Autodesk Inventor part; units mm, degrees
ref_plane "YZ Plane" through (0, 0, 0) normal (1, 0, 0) x (0, 1, 0)
ref_plane "XZ Plane" through (0, 0, 0) normal (0, 1, 0) x (-1, 0, 0)
ref_plane "XY Plane" through (0, 0, 0) normal (0, 0, 1) x (1, 0, 0)
sketch "Sketch1" plane through (0, 0, 0) normal (0, 0, 1) x (1, 0, 0)
  line L0 (0, 110) -> (110, 110)
  line L1 (110, 60) -> (110, 0)
  line L2 (110, 0) -> (0, 0)
  line L3 (0, 0) -> (0, 110)
  arc A0 (110, 110) -> (110, 60) centre (110, 85) ccw
  line L4 (73.8274, 98.9712) -> (73.8274, 60) construction
  line L5 (73.8274, 60) -> (92, 60) construction
  line L6 (73.8274, 98.9712) -> (92, 60)
  line L7 (92, 60) -> (73.8274, 98.9712) construction
  line L8 (73.8274, 98.9712) -> (71.1085, 97.7034)
  line L9 (71.1085, 97.7034) -> (89.2811, 58.7321)
  line L10 (89.2811, 58.7321) -> (92, 60)
  line L11 (0, 0) -> (10, 0)
  line L12 (10, 0) -> (10, -3)
  line L13 (10, -3) -> (0, -3)
  line L14 (0, -3) -> (0, 0)
  line L15 (30, 0) -> (30, -3)
  line L16 (20, 0) -> (30, 0)
  line L17 (20, -3) -> (20, 0)
  line L18 (30, -3) -> (20, -3)
  line L19 (50, 0) -> (50, -3)
  line L20 (40, 0) -> (50, 0)
  line L21 (40, -3) -> (40, 0)
  line L22 (50, -3) -> (40, -3)
  line L23 (70, 0) -> (70, -3)
  line L24 (60, 0) -> (70, 0)
  line L25 (60, -3) -> (60, 0)
  line L26 (70, -3) -> (60, -3)
  line L27 (90, 0) -> (90, -3)
  line L28 (80, 0) -> (90, 0)
  line L29 (80, -3) -> (80, 0)
  line L30 (90, -3) -> (80, -3)
  line L31 (110, 0) -> (110, -3)
  line L32 (100, 0) -> (110, 0)
  line L33 (100, -3) -> (100, 0)
  line L34 (110, -3) -> (100, -3)
  line L35 (10, 113) -> (10, 110)
  line L36 (0, 113) -> (10, 113)
  line L37 (0, 110) -> (0, 113)
  line L38 (10, 110) -> (0, 110)
  line L39 (30, 113) -> (30, 110)
  line L40 (20, 113) -> (30, 113)
  line L41 (20, 110) -> (20, 113)
  line L42 (30, 110) -> (20, 110)
  line L43 (50, 113) -> (50, 110)
  line L44 (40, 113) -> (50, 113)
  line L45 (40, 110) -> (40, 113)
  line L46 (50, 110) -> (40, 110)
  line L47 (70, 113) -> (70, 110)
  line L48 (60, 113) -> (70, 113)
  line L49 (60, 110) -> (60, 113)
  line L50 (70, 110) -> (60, 110)
  line L51 (90, 113) -> (90, 110)
  line L52 (80, 113) -> (90, 113)
  line L53 (80, 110) -> (80, 113)
  line L54 (90, 110) -> (80, 110)
  line L55 (110, 113) -> (110, 110)
  line L56 (100, 113) -> (110, 113)
  line L57 (100, 110) -> (100, 113)
  line L58 (110, 110) -> (100, 110)
  point P0 (0, 0)
  dimension "d1" = 110
  dimension "d2" = 110
  dimension "d3" = 110
  dimension "d4" = 25
  dimension "d6" = 18.1726
  dimension "d7" = 38.9712
  dimension "d8" = 18
  dimension "d9" = 3
  dimension "d12" = 3
  dimension "d13" = 10
  dimension "d16" = 20
  dimension "d19" = 113
extrude "Extrusion1" add sketch "Sketch1" along normal blind 3
sketch "Sketch2" plane through (0, 0, 3) normal (0, 0, 1) x (1, 0, 0)
  line L0 (0, 0) -> (-3, 0)
  line L1 (-3, 0) -> (-3, 10)
  line L2 (-3, 10) -> (0, 10)
  line L3 (0, 10) -> (0, 0)
  line L4 (0, 113) -> (0, -3) construction
  line L5 (90, 0) -> (100, 0) construction
  line L6 (0, 20) -> (-3, 20)
  line L7 (-3, 20) -> (-3, 30)
  line L8 (-3, 30) -> (0, 30)
  line L9 (0, 30) -> (0, 20)
  line L10 (0, 40) -> (-3, 40)
  line L11 (-3, 40) -> (-3, 50)
  line L12 (-3, 50) -> (0, 50)
  line L13 (0, 50) -> (0, 40)
  line L14 (0, 60) -> (-3, 60)
  line L15 (-3, 60) -> (-3, 70)
  line L16 (-3, 70) -> (0, 70)
  line L17 (0, 70) -> (0, 60)
  line L18 (0, 80) -> (-3, 80)
  line L19 (-3, 80) -> (-3, 90)
  line L20 (-3, 90) -> (0, 90)
  line L21 (0, 90) -> (0, 80)
  line L22 (0, 100) -> (-3, 100)
  line L23 (-3, 100) -> (-3, 110)
  line L24 (-3, 110) -> (0, 110)
  line L25 (0, 110) -> (0, 100)
  line L26 (113, 10) -> (113, 0)
  line L27 (113, 0) -> (110, 0)
  line L28 (110, 0) -> (110, 10)
  line L29 (110, 10) -> (113, 10)
  line L30 (0, 30) -> (0, 20)
  line L31 (0, 20) -> (-3, 20)
  line L32 (-3, 20) -> (-3, 30)
  line L33 (-3, 30) -> (0, 30)
  line L34 (113, 30) -> (113, 20)
  line L35 (113, 20) -> (110, 20)
  line L36 (110, 20) -> (110, 30)
  line L37 (110, 30) -> (113, 30)
  line L38 (0, 50) -> (0, 40)
  line L39 (0, 40) -> (-3, 40)
  line L40 (-3, 40) -> (-3, 50)
  line L41 (-3, 50) -> (0, 50)
  line L42 (113, 50) -> (113, 40)
  line L43 (113, 40) -> (110, 40)
  line L44 (110, 40) -> (110, 50)
  line L45 (110, 50) -> (113, 50)
  dimension "d22" = 3
  dimension "d23" = 10
  dimension "d26" = 20
  dimension "d33" = 113
  dimension "d36" = 20
extrude "Extrusion2" add sketch "Sketch2" against normal blind 3
properties part number "ParedPantalla"
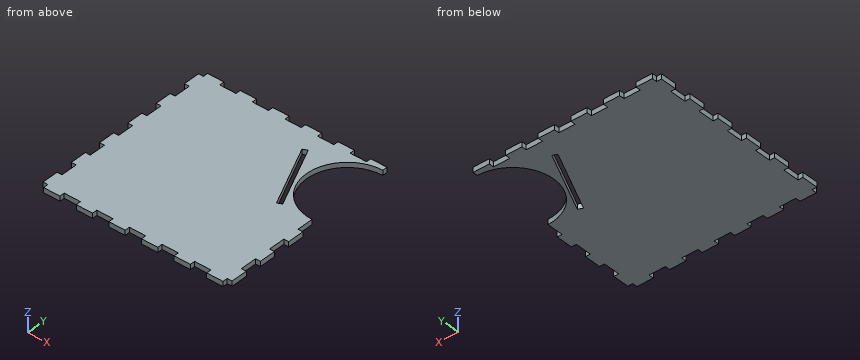
CAD build for the part. Positions are in the model's coordinates, mm. Round coordinates to 2 decimals unless told otherwise and drop trailing zeros. Order: outer loops, then holes, each group sorted by start corner. A loop starts at its lowest first (then second) coordinate and runs counter-clockwise, first axis right, second up.
Item 1: Saw through at A-A on x = 15. Write the cut outline in (y, z), then the cut area to 3 significant figures.
Item 2: Pin check, flat tips, straight feed: pin 1 (1.5 mm diameter, centred on y = -1.5, z = 1.5, fed in from -X); pin 2 (0.9 mm diameter, centred on y = 16, z = 1.5, fed in from +X); pin 3 (1 mm diameter, centred on x = 98, z = 1.5, fed in from -Y). Stop position of each tip, or through.
Item 3: Probe line 1 along Y through (x, z) = (87, 2.6); line 2 along X through (y, z) = (11.5, 2.3); line 3 along X through (y, z) = (67.5, 0.2). List the from-to ranges inside material, lowest first.
Reported:
1. outline: (0, 0) - (110, 0) - (110, 3) - (0, 3) - close
1. area: 330 mm2
2. pin 1: stops at x = 0
2. pin 2: stops at x = 110
2. pin 3: stops at y = 0
3. line 1: y = -3 to 63.62, 70.72 to 75.2, 94.8 to 113
3. line 2: x = 0 to 110
3. line 3: x = -3 to 85.19, 88.5 to 92.15
